```python
from build123d import *

# Parameters (mm, degrees)
F0_W     = 50
F0_H     = 85
F0_R     = 2.5
F0_R_2   = 2
F0_H_2   = 30
F0_R_3   = 9.6
F1_DEPTH = 6
F2_DEPTH = 2
F3_DEPTH = 17
F0_R_4   = 8.5
F4_DEPTH = 10


with BuildPart() as f1:
    # F0 (on Top) → F1 (new body)
    with BuildSketch(Plane.XY):
        with Locations((25, 42.5)):
            Rectangle(F0_W, F0_H)
        with Locations((7, 7)):
            Circle(F0_R, mode=Mode.SUBTRACT)
        with Locations((43, 7)):
            Circle(F0_R, mode=Mode.SUBTRACT)
        Polygon((35.5, 5), (15, 5), (15, 13), (15, 53), (15, 61), (35.5, 61), (35.5, 53), (35.5, 13), align=None, mode=Mode.SUBTRACT)
        with Locations((7, 63)):
            Circle(F0_R, mode=Mode.SUBTRACT)
        with Locations((43, 63)):
            Circle(F0_R, mode=Mode.SUBTRACT)
        Polygon((15, 61), (15, 53), (24.25, 53), (24.25, 59), (26.25, 59), (26.25, 53), (35.5, 53), (35.5, 61), align=None)
        with Locations((20.25, 57)):
            Circle(F0_R_2, mode=Mode.SUBTRACT)
        with Locations((30.25, 57)):
            Circle(F0_R_2, mode=Mode.SUBTRACT)
        Polygon((15, 13), (15, 5), (35.5, 5), (35.5, 13), (26.25, 13), (26.25, 7), (24.25, 7), (24.25, 13), align=None)
        with Locations((20.25, 9)):
            Circle(F0_R_2, mode=Mode.SUBTRACT)
        with Locations((30.25, 9)):
            Circle(F0_R_2, mode=Mode.SUBTRACT)
        with Locations((25, 100)):
            Rectangle(F0_W, F0_H_2)
        with Locations((25, 104)):
            Circle(F0_R_3, mode=Mode.SUBTRACT)
    extrude(amount=-F1_DEPTH)

    # F0 (on Top) → F2 (cut)
    with BuildSketch(Plane.XY):
        Polygon((15, 61), (15, 53), (24.25, 53), (24.25, 59), (26.25, 59), (26.25, 53), (35.5, 53), (35.5, 61), align=None)
        with Locations((20.25, 57)):
            Circle(F0_R_2, mode=Mode.SUBTRACT)
        with Locations((30.25, 57)):
            Circle(F0_R_2, mode=Mode.SUBTRACT)
        Polygon((15, 13), (15, 5), (35.5, 5), (35.5, 13), (26.25, 13), (26.25, 7), (24.25, 7), (24.25, 13), align=None)
        with Locations((20.25, 9)):
            Circle(F0_R_2, mode=Mode.SUBTRACT)
        with Locations((30.25, 9)):
            Circle(F0_R_2, mode=Mode.SUBTRACT)
    extrude(amount=-F2_DEPTH, mode=Mode.SUBTRACT)

    # F0 (on Top) → F3 (join)
    with BuildSketch(Plane.XY):
        with Locations((25, 100)):
            Rectangle(F0_W, F0_H_2)
        with Locations((25, 104)):
            Circle(F0_R_3, mode=Mode.SUBTRACT)
    extrude(amount=F3_DEPTH)

    # F0 (on Top) → F4 (join)
    with BuildSketch(Plane.XY):
        with Locations((25, 104)):
            Circle(F0_R_3)
        with Locations((25, 104)):
            Circle(F0_R_4, mode=Mode.SUBTRACT)
    extrude(amount=F4_DEPTH)


solid = f1.part
```
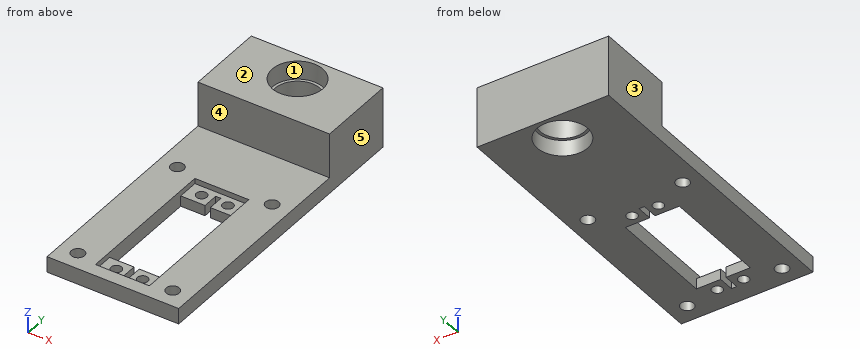
Source: CAD feature listing. Evaluate the final solid. Frame: model axes, mm. Face numbers are marked on the shaded views. A direction names the side the tool comes from. Give positions to 0.01 mm unless a question says otherwise; leave off trailing zeros. Write each loop counter-clockwise with the first axis right and the second up, starting at its lowest first coordinate (ties: lowest second). Pieces come first, ordered by that corner, then holes. Notation, with made-up numbers: (64.5, 24.5) - (107.5, 24.5) arc R22 ccw to (107.5, 30.5) - close; hole circle Ø1 at (52, 38.25). An arc over 180 degrees is marked (long way). One line per item, written item: value. Start each with the question number.
Q1. Section query D-D, the plane y = 25.5. Return the cut outline in (x, z).
Q2. Draft query along X for the marked faces 1, 2 and 3. Return one class per face: +X half, -X half, draft (parallel to the pull), parting line (faces both ways), or undercut.
Q3. Section query C-C, the plane z = -3.5. Count the separate pieces of the cut face and the enclosed holes in it, then the cut area to 3 significant figures.
Q4. Set-up query: the marked faces 4 and 5. Return all of +Z, -Z, +X, -X, +Y, -Y with unobstructed straight access to the full face (end or side cutting, diameter ignored); none if empty.
Q5. Material intervals for probe 1 along Y at (x, z) = (9.5, 5.5); probe 2 along Z at (x, y) = (30, 77); probe 3 along X at (y, z) = (35, -2), sorted ascending. Write a range as from..to.
Q6. First-contact query: pin 1 Ø1 at (x, y) = (29.5, 14.5) entering from +Z; pin 2 Ø2 at (x, y) = (36, 56.5) entering from +Z; pin 3 Ø6.5 at (x, y) = (26.5, 8.5) entering from +Z; pin 4 Ø1 at (x, z) = (25, 10) entering from -Y. Flat tips, straight axial feed; report the tip coordinate or a pass-through.
Q7. Section query B-B, the plane y = 57. Return the cut outline in (x, z), then the cut area to 3 significant figures.
Q8. Section query A-A, the plane x = 7. Return the cut outline in (y, z).
Answer:
1. outline: (0, -6) - (15, -6) - (15, 0) - (0, 0) - close; (35.5, -6) - (50, -6) - (50, 0) - (35.5, 0) - close
2. face 1: undercut
2. face 2: draft
2. face 3: -X half
3. separate pieces: 1
3. enclosed holes: 10
3. area: 4,490 mm2
4. face 4: +Z, +X, -X, -Y
4. face 5: +Z, -Z, +X, +Y, -Y
5. probe 1: y = 85..115
5. probe 2: z = -6..0
5. probe 3: x = 0..15, 35.5..50
6. pin 1: passes through
6. pin 2: stops at z = 0
6. pin 3: stops at z = -2
6. pin 4: stops at y = 85
7. outline: (0, -6) - (18.25, -6) - (18.25, -2) - (15, -2) - (15, 0) - (0, 0) - close; (22.25, -6) - (24.25, -6) - (24.25, -2) - (22.25, -2) - close; (26.25, -6) - (28.25, -6) - (28.25, -2) - (26.25, -2) - close; (32.25, -6) - (50, -6) - (50, 0) - (35.5, 0) - (35.5, -2) - (32.25, -2) - close
7. area: 219 mm2
8. outline: (0, -6) - (4.5, -6) - (4.5, 0) - (0, 0) - close; (9.5, -6) - (60.5, -6) - (60.5, 0) - (9.5, 0) - close; (65.5, -6) - (115, -6) - (115, 17) - (85, 17) - (85, 0) - (65.5, 0) - close
